Geometry: final body of the model. Coordinates: model frame, mm. A direction names the side the tool comes from. Give positions to 0.01 mm unless a question says otherwise; leave off trailing zeros. Loops run counter-clockwise (first coordinate to the right, second up) from the corner with the lowest first, then second, coordinate; pieces in that order, holes last. Notation, with made-up numbers: (50.5, -9) -> (56.5, -9) arc R6 ccw to (56.5, 0) -> close; hole circle Ø5 at (27.5, -29.75). An arc over 180 degrees is marked (long way). Answer in a Markdown table with one row per item. Add a question column.
1) Section query D-D (y = -14.5). Return the cut outline in (x, z).
2) Access query for faces 1 (the flat face through (-31.826, -25, 17)), 2 (the flat face through (-26.756, -7, 22)). Directions: +Z, -Z, +X, -X, +Y, -Y. A direction counts if a zero-diameter tool reaches every point of the face in a straight line with its end or side. Return the directions, or none.
3) Section query C-C (y = -5). Return the cut outline in (x, z), plus the area to 3 significant figures.
4) Draft query along Z for faces 3 (the flat face through (-27, 0, 13)), 4 (the flat face through (-27, -25, 10.631)), 5 (the flat face through (-27, -25, 23.331)), 6 (the cylindrical face through (-29.93, -25.76, 14.66)). Return one class per face: +Z half, -Z half, draft (parallel to the pull), parting line (faces both ways), or undercut.
5) Section query A-A (z = 15.25). Return the cut outline in (x, y), plus the area to 3 significant figures.
6) Line query: line 1 (X direction, y = -2.5, z = 17); line 2 (Z direction, x = -28.75, y = -6.5); line 3 (Z direction, x = -29.75, y = -8). Output: solid intervals per line, ascending. Write a range as from..to.
7) Section query B-B (x = -28.5). Return the cut outline in (y, z), plus the area to 3 significant figures.
```python
from build123d import *

# Parameters (mm, degrees)
F0_W     = 10.16
F0_H     = 12.7
F1_DEPTH = 50.8
F2_R     = 3.81
F3_DEPTH = 76.2
F4_W     = 0.254
F4_H     = 10.16
F5_DEPTH = 2.2606


with BuildPart() as f1:
    # F0 (on Front) → F1 (new body)
    with BuildSketch(Plane.XZ):
        with Locations((-26.745969, 16.98054)):
            Rectangle(F0_W, F0_H)
    extrude(amount=F1_DEPTH)

    # F2 (on face) → F3 (cut)
    with BuildSketch(Plane.XZ.offset(50.8)):
        with Locations((-26.909839, 16.98054)):
            Circle(F2_R)
    extrude(amount=-F3_DEPTH, mode=Mode.SUBTRACT)

    # F4 (on face) → F5 (cut)
    with BuildSketch(Plane.XY.offset(23.33054)):
        with Locations((-26.883121, -7.359638)):
            Rectangle(F4_W, F4_H)
    extrude(amount=-F5_DEPTH, mode=Mode.SUBTRACT)


solid = f1.part
```
Evaluation:
| question | item | result |
|---|---|---|
| 1 | outline | (-31.83, 10.63) -> (-21.67, 10.63) -> (-21.67, 23.33) -> (-31.83, 23.33) -> close; hole circle Ø7.62 at (-26.91, 16.98) |
| 2 | face 1 | +Z, -Z, -X, +Y, -Y |
| 2 | face 2 | +Z |
| 3 | outline | (-31.83, 10.63) -> (-21.67, 10.63) -> (-21.67, 23.33) -> (-26.76, 23.33) -> (-26.76, 21.07) -> (-27.01, 21.07) -> (-27.01, 23.33) -> (-31.83, 23.33) -> close; hole circle Ø7.62 at (-26.91, 16.98) |
| 3 | area | 82.9 mm² |
| 4 | face 3 | draft |
| 4 | face 4 | -Z half |
| 4 | face 5 | +Z half |
| 4 | face 6 | undercut |
| 5 | outline | (-31.83, -50.8) -> (-30.3, -50.8) -> (-30.3, 0) -> (-31.83, 0) -> close; (-23.52, -50.8) -> (-21.67, -50.8) -> (-21.67, 0) -> (-23.52, 0) -> close |
| 5 | area | 171 mm² |
| 6 | line 1 | -31.83..-30.72, -23.1..-21.67 |
| 6 | line 2 | 10.63..13.64, 20.32..23.33 |
| 6 | line 3 | 10.63..14.44, 19.52..23.33 |
| 7 | outline | (-50.8, 10.63) -> (0, 10.63) -> (0, 13.52) -> (-50.8, 13.52) -> close; (-50.8, 20.44) -> (0, 20.44) -> (0, 23.33) -> (-50.8, 23.33) -> close |
| 7 | area | 293 mm² |
